The figure shows three views and two pictorial views of one solid part (mm, origin at its lowest corner). Answer the questions. A direction names the side the tool comes from. Give positions to 0.01 mm unless a question says otherwise; leave off trailing zeros. Write each loop counter-clockwise with the first axis right and the second up, starting at its lowest first coordinate (ties: lowest second). Pieces come first, ordered by that corner, then holes. Notation, with made-up numbers: (84.25, 67.25) -> (127.25, 67.25) arc R19 cw to (127.25, 93.25) -> close; hole circle Ø4 at (70, -36.5). An arc over 180 degrees is marked (long way). Write item = value, one per line. Start each with the question number.
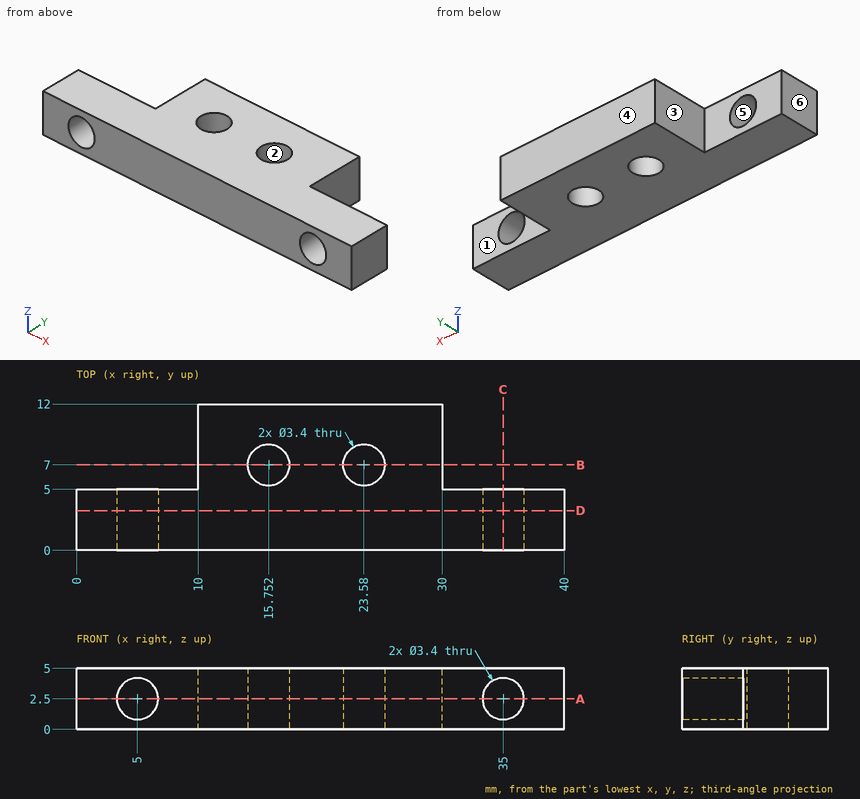
(1) A cutting plane is placed at D-D, the plane y = 3.25. Write down the section's boundary in (x, z).
(2) A cutting plane is placed at A-A, the plane z = 2.5. Write down the section's boundary in (x, y), then the cut area to 3 significant figures.
(3) Find the intervals of material crossed by line 1 along Z through (x, y) = (35, 1.2); line 2 along Y through (x, z) = (3, 1.35); line 3 along X through (y, z) = (7.25, 1.5), in increasing order.
(4) For the marked faces 1, 2 and 3, determine the directions among +Z, -Z, +X, -X, +Y, -Y from which every point of the face is accessible in a straight line to the end or side of a thin tool.
(5) A cutting plane is placed at C-C, the plane x = 35. Write down the section's boundary in (y, z).
(6) Each of these flat-tipped pins is pushed along its axis until it touches: pin 1 (2 mm diameter, centred on x = 28, z = 0.5, fed in from -Y); pin 2 (1 mm diameter, centred on y = 6.5, z = 3.5, fed in from -X); pin 3 (2.5 mm diameter, centred on x = 36.5, z = 3.5, fed in from +Y); pin 4 (1.5 mm diameter, centred on y = 9.5, z = 3.5, fed in from +X). Where does it stop, or does it pass through?
(7) Determine the mould class of the marked faces 4, 5 and 6 for opening direction X: pulls with the +X half, pulls with the -X half, needs draft (parallel to the pull), parting line crosses it, or undercut.
(8) A cutting plane is placed at B-B, the plane y = 7. Write down the section's boundary in (x, z), then the cut area to 3 significant figures.
Results list:
q1.outline = (0, 0) -> (40, 0) -> (40, 5) -> (0, 5) -> close; hole circle Ø3.4 at (5, 2.5); hole circle Ø3.4 at (35, 2.5)
q2.outline = (0, 0) -> (3.3, 0) -> (3.3, 5) -> (0, 5) -> close; (6.7, 0) -> (33.3, 0) -> (33.3, 5) -> (30, 5) -> (30, 12) -> (10, 12) -> (10, 5) -> (6.7, 5) -> close; (36.7, 0) -> (40, 0) -> (40, 5) -> (36.7, 5) -> close; hole circle Ø3.4 at (15.75, 7); hole circle Ø3.4 at (23.58, 7)
q2.area = 288 mm²
q3.line_1 = 0 to 0.8, 4.2 to 5
q3.line_2 = 0 to 5
q3.line_3 = 10 to 14.07, 17.43 to 21.9, 25.26 to 30
q4.face_1 = +Z, -Z, +X, +Y
q4.face_2 = +Z, -Z
q4.face_3 = +Z, -Z, -X, +Y
q5.outline = (0, 0) -> (5, 0) -> (5, 0.8) -> (0, 0.8) -> close; (0, 4.2) -> (5, 4.2) -> (5, 5) -> (0, 5) -> close
q6.pin_1 = 0
q6.pin_2 = 10
q6.pin_3 = 5
q6.pin_4 = 30
q7.face_4 = needs draft
q7.face_5 = undercut
q7.face_6 = pulls with the -X half
q8.outline = (10, 0) -> (14.05, 0) -> (14.05, 5) -> (10, 5) -> close; (17.45, 0) -> (21.88, 0) -> (21.88, 5) -> (17.45, 5) -> close; (25.28, 0) -> (30, 0) -> (30, 5) -> (25.28, 5) -> close
q8.area = 66.0 mm²
